For this review, take the finished solid that the model builds, in its own axes (mm). Face numbers are marked on the shaded views. A direction names the side the tool comes from. Coordinates: 2 decimals unless noted, no trailing zeros. Loops run counter-clockwise (first coordinate to the right, second up) from the corner with the lowest first, then second, coordinate; pieces in that order, holes last. Notation, with made-up numbers: (9.25, 67) - (27.25, 67) arc R24 cw to (27.25, 103) - close; hole circle Ø3 at (-29, 75). An arc over 180 degrees is marked (long way). Answer as a JSON object with one key per item and string values. Group by question number.
Item 1: Tool access review of the marked faces 1, 2 and 3: name each direction out of +Z, -Z, +X, -X, +Y, -Y from which nothing blocks a thin tool from reaching the whole face with its end or side.
Item 2: We need section B-B (x = 7.25). Give the boundary of the cut face in (y, z).
Item 3: To check wall thickness, follow line 1 (Z direction, x = 13.25, y = 6.5); line 2 (Y direction, x = 19, z = 3.5); line 3 (Y direction, x = 0.5, z = 14). State the ranges of each line that lie inside material, in increasing order.
Item 4: We need section A-A (z = 8.5). State how many separate pieces and enclosed holes the cut face has, then the cut area to 3 significant figures.
Item 5: We need section C-C (y = 11.5). Give the boundary of the cut face in (x, z).
Item 6: We need section D-D (z = 10.5). Give the boundary of the cut face in (x, y).
Item 7: Mouldability with a two-part tool opening along Z and no side actions: class the marked faces 4, 5 and 6 as released by +Z, released by -Z, zero draft, split by the parting line, or undercut.
Item 8: Clearance check with flat-ended pins moving along their axes: pin 1 (6 mm diameter, centred on y = 11.5, z = 6, fed in from +X); pin 2 (4 mm diameter, centred on x = 7, z = 12.5, fed in from -Y); pin 3 (0.8 mm diameter, centred on y = -0.5, z = 8, fed in from -X); pin 4 (8 mm diameter, centred on x = 10, y = 17.5, fed in from -Z). State where each tip first meets the part, or that it passes through.
from build123d import *

# Parameters (mm, degrees)
BOSS_EXTRUDE1_DEPTH = 17
SKETCH2_W           = 17
SKETCH2_H           = 17
CUT_EXTRUDE1_DEPTH  = 13
CUT_EXTRUDE2_DEPTH  = 13
SKETCH6_W           = 3.5
SKETCH6_H           = 1.5
BOSS_EXTRUDE2_DEPTH = 1
FILLET1_R           = 0.75
SKETCH7_W           = 1.5
SKETCH7_H           = 3.5
BOSS_EXTRUDE3_DEPTH = 1
FILLET2_R           = 0.75
CUT_EXTRUDE3_DEPTH  = 10


with BuildPart() as part:
    # Sketch1 → Boss-Extrude1 (new body)
    with BuildSketch(Plane.XY):
        Polygon((0, 0), (0, 20), (3.029437252, 20), (20, 3.029437252), (20, 0), align=None)
    extrude(amount=BOSS_EXTRUDE1_DEPTH)

    # Sketch2 → Cut-Extrude1 (cut)
    with BuildSketch(Plane.XY.offset(2)):
        with Locations((11.5, 11.5)):
            Rectangle(SKETCH2_W, SKETCH2_H)
    extrude(amount=CUT_EXTRUDE1_DEPTH, mode=Mode.SUBTRACT)

    # Sketch3 → Cut-Extrude2 (cut)
    with BuildSketch(Plane(origin=(0, 0, 0), x_dir=(1, 0, 0), z_dir=(0, 1, 0))):
        with BuildLine():
            Line((8.5, -5.25), (12, -5.25))
            ThreePointArc((12, -5.25), (15.25, -8.5), (12, -11.75))
            Line((12, -11.75), (8.5, -11.75))
            ThreePointArc((8.5, -11.75), (5.25, -8.5), (8.5, -5.25))
        make_face()
    extrude(amount=CUT_EXTRUDE2_DEPTH, mode=Mode.SUBTRACT)

    # Sketch6 → Boss-Extrude2 (add)
    with BuildSketch(Plane(origin=(0, 0, 0), x_dir=(0, 0, -1), z_dir=(1, 0, 0))):
        with Locations((-8.25, 18.25)):
            Rectangle(SKETCH6_W, SKETCH6_H)
        with Locations((-8.25, 2.75)):
            Rectangle(SKETCH6_W, SKETCH6_H)
    extrude(amount=-BOSS_EXTRUDE2_DEPTH)

    # Fillet1
    fillet1_edges = [part.edges().sort_by_distance(p)[0] for p in [
        (-0.5, 2, 6.5),
        (-0.5, 17.5, 6.5),
        (-0.5, 2, 10),
        (-0.5, 3.5, 10),
        (-0.5, 3.5, 6.5),
        (-0.5, 17.5, 10),
        (-0.5, 19, 10),
        (-0.5, 19, 6.5),
    ]]
    fillet(fillet1_edges, radius=FILLET1_R - 0.0001)  # a hair under: the kernel refuses the full size

    # Sketch7 → Boss-Extrude3 (add)
    with BuildSketch(Plane(origin=(0, 0, 0), x_dir=(1, 0, 0), z_dir=(0, 1, 0))):
        with Locations((2.75, -8.25)):
            Rectangle(SKETCH7_W, SKETCH7_H)
        with Locations((18.25, -8.25)):
            Rectangle(SKETCH7_W, SKETCH7_H)
    extrude(amount=-BOSS_EXTRUDE3_DEPTH)

    # Fillet2
    fillet2_edges = [part.edges().sort_by_distance(p)[0] for p in [
        (3.5, -0.5, 6.5),
        (2, -0.5, 6.5),
        (2, -0.5, 10),
        (3.5, -0.5, 10),
        (17.5, -0.5, 10),
        (19, -0.5, 10),
        (17.5, -0.5, 6.5),
        (19, -0.5, 6.5),
    ]]
    fillet(fillet2_edges, radius=FILLET2_R - 0.0001)  # a hair under: the kernel refuses the full size

    # Sketch8 → Cut-Extrude3 (cut)
    with BuildSketch(Plane(origin=(0, 0, 0), x_dir=(0, 0, -1), z_dir=(1, 0, 0))):
        with BuildLine():
            Line((-11.75, 8.5), (-11.75, 12))
            ThreePointArc((-11.75, 12), (-8.5, 15.25), (-5.25, 12))
            Line((-5.25, 12), (-5.25, 8.5))
            ThreePointArc((-5.25, 8.5), (-8.5, 5.25), (-11.75, 8.5))
        make_face()
    extrude(amount=CUT_EXTRUDE3_DEPTH, mode=Mode.SUBTRACT)


solid = part.part
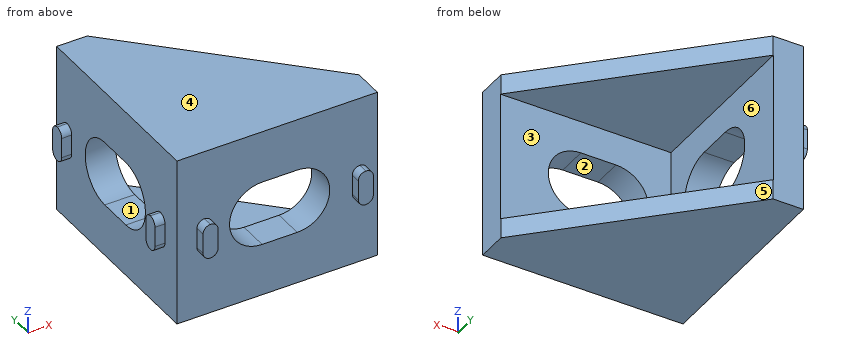
Check sheet entries:
{
 "1": {"face 1": "+X, -X", "face 2": "+Y, -Y", "face 3": "+X, +Y"},
 "2": {"outline": "(0, 0) - (15.78, 0) - (15.78, 2) - (3, 2) - (3, 5.5) - (0, 5.5) - close; (0, 11.5) - (3, 11.5) - (3, 15) - (15.78, 15) - (15.78, 17) - (0, 17) - close"},
 "3": {"line 1": "z = 0 to 2, 15 to 17", "line 2": "y = 0 to 3", "line 3": "y = 0 to 20"},
 "4": {"separate pieces": "3", "enclosed holes": "0", "area": "57.0 mm2"},
 "5": {"outline": "(0, 0) - (11.53, 0) - (11.53, 2) - (3, 2) - (3, 5.25) - (0, 5.25) - close; (0, 11.75) - (3, 11.75) - (3, 15) - (11.53, 15) - (11.53, 17) - (0, 17) - close"},
 "6": {"outline": "(0, 0) - (5.94, 0) - (5.94, 3) - (3, 3) - (3, 5.94) - (0, 5.94) - close; (0, 14.56) - (3, 14.56) - (3, 20) - (0, 20) - close; (14.56, 0) - (20, 0) - (20, 3) - (14.56, 3) - close"},
 "7": {"face 4": "released by +Z", "face 5": "zero draft", "face 6": "undercut"},
 "8": {"pin 1": "stops at x = 3", "pin 2": "stops at y = 0", "pin 3": "stops at x = 2", "pin 4": "stops at z = 0"}
}
